Source: three-view drawing plus pictorial views. Frame: mm from the lowest corner of the part. A direction names the side the tool comes from. Give positions to 0.01 mm unless a question says otherwise; leave off trailing zeros. Order: outer loops, then holes, each group sorted by start corner. A loop starts at its lowest first (then second) coordinate and runs counter-clockwise, first axis right, second up. Notation, with made-up numbers: (25.25, 36.5) -> (53.25, 36.5) arc R24 cw to (53.25, 74.5) -> close; hole circle Ø2 at (-14, 41.25). An arc over 180 degrees is marked (long way). Answer in a Markdown table with one row per item. Add a question column.
Q1. Cut plane B-B on y = 21.75. Return the cut outline in (x, z) (1 decimal).
Q2. Cut plane A-A on x = 7.7. Return the cut outline in (y, z) (1 decimal).
Q3. Cut plane C-C on z = 22.75. Return the cut outline in (x, y) (1 decimal).
Q4. Cut plane D-D on x = 2. Return the cut outline in (y, z), and give its area (3 significant figures).
Q5. Contact query for flat-ended pins moving along their axis: P1, Ø5, axis at x = 17.7, z = 17.7, coming from the +Y side (1 decimal); P2, Ø2.5, axis at y = 8.29, z = 18.7, coming from the -X side; P3, Ø10, axis at x = 5.5, z = 12, coming from the -Y side; P4, Ø5.5, axis at x = 12.5, z = 9, coming from the +Y side (1 decimal). Output: stop coordinate, or through.
Q6. Set-up query: the marked faces 5 and 6. Return all of +Z, -Z, +X, -X, +Y, -Y with unobstructed straight access to the full face (end or side cutting, diameter ignored); none if empty.
Q7. Line query: line 1 along Z through (x, y) = (17.7, 0.2); line 2 along Y through (x, z) = (24.45, 18.7). Output: solid intervals per line, ascending. Write a range as from..to.
Q8. Pull-direction query (X, two-part tool) for the marked faces 1, 2, 3 and 4; classes: +X half, -X half, draft (parallel to the pull), parting line (faces both ways), or undercut.
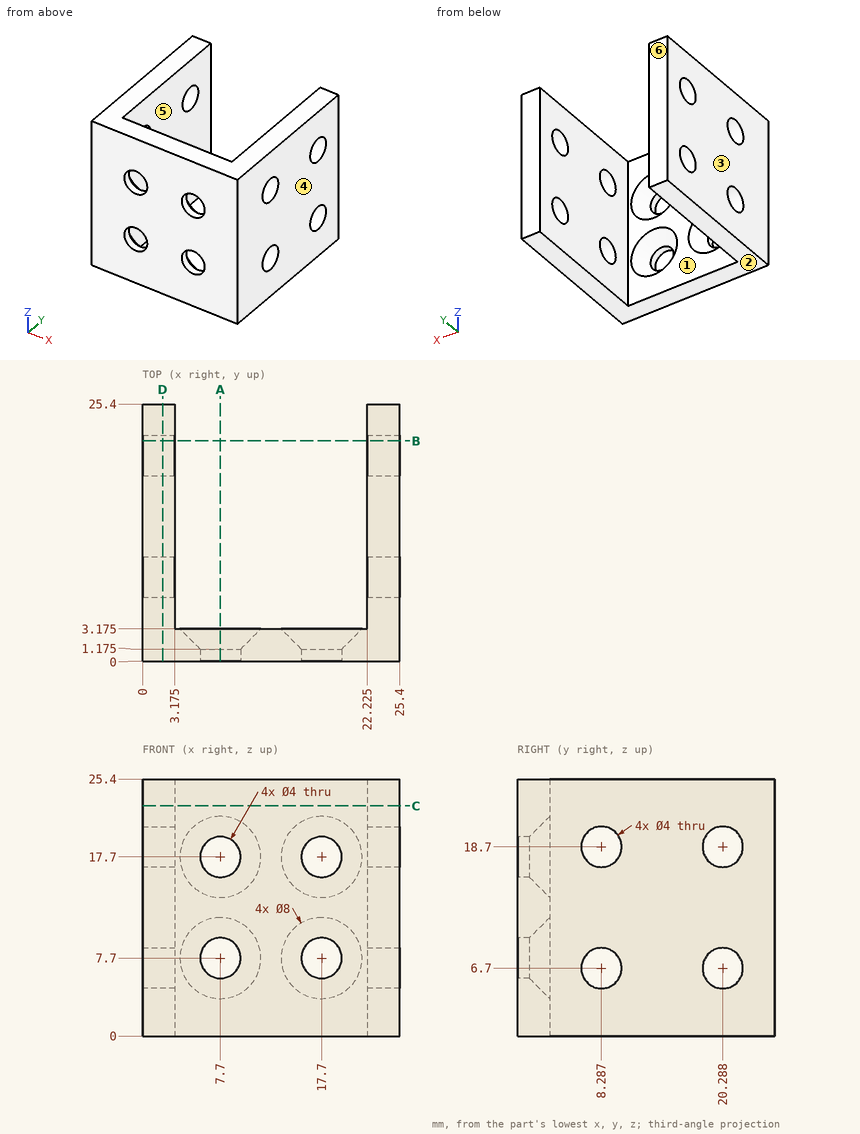
Completed:
| question | item | result |
|---|---|---|
| 1 | outline | (0, 0) -> (3.2, 0) -> (3.2, 5.3) -> (0, 5.3) -> close; (0, 8.1) -> (3.2, 8.1) -> (3.2, 17.3) -> (0, 17.3) -> close; (0, 20.1) -> (3.2, 20.1) -> (3.2, 25.4) -> (0, 25.4) -> close; (22.2, 0) -> (25.4, 0) -> (25.4, 5.3) -> (22.2, 5.3) -> close; (22.2, 8.1) -> (25.4, 8.1) -> (25.4, 17.3) -> (22.2, 17.3) -> close; (22.2, 20.1) -> (25.4, 20.1) -> (25.4, 25.4) -> (22.2, 25.4) -> close |
| 2 | outline | (0, 0) -> (3.2, 0) -> (3.2, 3.7) -> (1.2, 5.7) -> (0, 5.7) -> close; (0, 9.7) -> (1.2, 9.7) -> (3.2, 11.7) -> (3.2, 13.7) -> (1.2, 15.7) -> (0, 15.7) -> close; (0, 19.7) -> (1.2, 19.7) -> (3.2, 21.7) -> (3.2, 25.4) -> (0, 25.4) -> close |
| 3 | outline | (0, 0) -> (25.4, 0) -> (25.4, 25.4) -> (22.2, 25.4) -> (22.2, 3.2) -> (3.2, 3.2) -> (3.2, 25.4) -> (0, 25.4) -> close |
| 4 | outline | (0, 0) -> (25.4, 0) -> (25.4, 25.4) -> (0, 25.4) -> close; hole circle Ø4 at (8.29, 6.7); hole circle Ø4 at (8.29, 18.7); hole circle Ø4 at (20.29, 6.7); hole circle Ø4 at (20.29, 18.7) |
| 4 | area | 595 mm² |
| 5 | P1 | stops at y = 1.7 |
| 5 | P2 | passes through |
| 5 | P3 | stops at y = 0 |
| 5 | P4 | stops at y = 3.2 |
| 6 | face 5 | +Z, -Z, +Y |
| 6 | face 6 | +Z, -Z, +X, -X, +Y |
| 7 | line 1 | z = 0..5.7, 9.7..15.7, 19.7..25.4 |
| 7 | line 2 | y = 0..6.29, 10.29..18.29, 22.29..25.4 |
| 8 | face 1 | undercut |
| 8 | face 2 | draft |
| 8 | face 3 | -X half |
| 8 | face 4 | +X half |
